from build123d import *

# Parameters (mm, degrees)
SKETCH_3_R      = 3.4
EXTRUDE_1_DEPTH = 2554


with BuildPart() as part:
    # 草图3 → 凸台-拉伸1 (new body)
    with BuildSketch(Plane(origin=(0, 0, 0), x_dir=(1, 0, 0), z_dir=(0, 1, 0))):
        with BuildLine():
            Line((-15, -12.5), (-15, -5.4))
            ThreePointArc((-15, -5.4), (-14.941421356, -5.258578644), (-14.8, -5.2))
            Line((-14.8, -5.2), (-14.4, -5.2))
            ThreePointArc((-14.4, -5.2), (-14.258578644, -5.141421356), (-14.2, -5))
            Line((-14.2, -5), (-14.2, -4.3))
            ThreePointArc((-14.2, -4.3), (-14.141421356, -4.158578644), (-14, -4.1))
            Line((-14, -4.1), (-13.2, -4.1))
            Line((-13.2, -4.1), (-13.2, -8.25))
            Line((-13.2, -8.25), (-9.522792206, -8.25))
            Line((-9.522792206, -8.25), (-5.8, -4.527207794))
            Line((-5.8, -4.527207794), (-5.8, 4.527207794))
            Line((-5.8, 4.527207794), (-9.522792206, 8.25))
            Line((-9.522792206, 8.25), (-13.2, 8.25))
            Line((-13.2, 8.25), (-13.2, 4.1))
            Line((-13.2, 4.1), (-14, 4.1))
            ThreePointArc((-14, 4.1), (-14.141421356, 4.158578644), (-14.2, 4.3))
            Line((-14.2, 4.3), (-14.2, 5))
            ThreePointArc((-14.2, 5), (-14.258578644, 5.141421356), (-14.4, 5.2))
            Line((-14.4, 5.2), (-14.8, 5.2))
            ThreePointArc((-14.8, 5.2), (-14.941421356, 5.258578644), (-15, 5.4))
            Line((-15, 5.4), (-15, 12.5))
            ThreePointArc((-15, 12.5), (-14.267766953, 14.267766953), (-12.5, 15))
            Line((-12.5, 15), (-5.4, 15))
            ThreePointArc((-5.4, 15), (-5.258578644, 14.941421356), (-5.2, 14.8))
            Line((-5.2, 14.8), (-5.2, 14.4))
            ThreePointArc((-5.2, 14.4), (-5.141421356, 14.258578644), (-5, 14.2))
            Line((-5, 14.2), (-4.3, 14.2))
            ThreePointArc((-4.3, 14.2), (-4.158578644, 14.141421356), (-4.1, 14))
            Line((-4.1, 14), (-4.1, 13.2))
            Line((-4.1, 13.2), (-8.25, 13.2))
            Line((-8.25, 13.2), (-8.25, 9.522792206))
            Line((-8.25, 9.522792206), (-4.527207794, 5.8))
            Line((-4.527207794, 5.8), (4.527207794, 5.8))
            Line((4.527207794, 5.8), (8.25, 9.522792206))
            Line((8.25, 9.522792206), (8.25, 13.2))
            Line((8.25, 13.2), (4.1, 13.2))
            Line((4.1, 13.2), (4.1, 14))
            ThreePointArc((4.1, 14), (4.158578644, 14.141421356), (4.3, 14.2))
            Line((4.3, 14.2), (5, 14.2))
            ThreePointArc((5, 14.2), (5.141421356, 14.258578644), (5.2, 14.4))
            Line((5.2, 14.4), (5.2, 14.8))
            ThreePointArc((5.2, 14.8), (5.258578644, 14.941421356), (5.4, 15))
            Line((5.4, 15), (12.5, 15))
            ThreePointArc((12.5, 15), (14.267766953, 14.267766953), (15, 12.5))
            Line((15, 12.5), (15, 5.4))
            ThreePointArc((15, 5.4), (14.941421356, 5.258578644), (14.8, 5.2))
            Line((14.8, 5.2), (14.4, 5.2))
            ThreePointArc((14.4, 5.2), (14.258578644, 5.141421356), (14.2, 5))
            Line((14.2, 5), (14.2, 4.3))
            ThreePointArc((14.2, 4.3), (14.141421356, 4.158578644), (14, 4.1))
            Line((14, 4.1), (13.2, 4.1))
            Line((13.2, 4.1), (13.2, 8.25))
            Line((13.2, 8.25), (9.522792206, 8.25))
            Line((9.522792206, 8.25), (5.8, 4.527207794))
            Line((5.8, 4.527207794), (5.8, -4.527207794))
            Line((5.8, -4.527207794), (9.522792206, -8.25))
            Line((9.522792206, -8.25), (13.2, -8.25))
            Line((13.2, -8.25), (13.2, -4.1))
            Line((13.2, -4.1), (14, -4.1))
            ThreePointArc((14, -4.1), (14.141421356, -4.158578644), (14.2, -4.3))
            Line((14.2, -4.3), (14.2, -5))
            ThreePointArc((14.2, -5), (14.258578644, -5.141421356), (14.4, -5.2))
            Line((14.4, -5.2), (14.8, -5.2))
            ThreePointArc((14.8, -5.2), (14.941421356, -5.258578644), (15, -5.4))
            Line((15, -5.4), (15, -12.5))
            ThreePointArc((15, -12.5), (14.267766953, -14.267766953), (12.5, -15))
            Line((12.5, -15), (5.4, -15))
            ThreePointArc((5.4, -15), (5.258578644, -14.941421356), (5.2, -14.8))
            Line((5.2, -14.8), (5.2, -14.4))
            ThreePointArc((5.2, -14.4), (5.141421356, -14.258578644), (5, -14.2))
            Line((5, -14.2), (4.3, -14.2))
            ThreePointArc((4.3, -14.2), (4.158578644, -14.141421356), (4.1, -14))
            Line((4.1, -14), (4.1, -13.2))
            Line((4.1, -13.2), (8.25, -13.2))
            Line((8.25, -13.2), (8.25, -9.522792206))
            Line((8.25, -9.522792206), (4.527207794, -5.8))
            Line((4.527207794, -5.8), (-4.527207794, -5.8))
            Line((-4.527207794, -5.8), (-8.25, -9.522792206))
            Line((-8.25, -9.522792206), (-8.25, -13.2))
            Line((-8.25, -13.2), (-4.1, -13.2))
            Line((-4.1, -13.2), (-4.1, -14))
            ThreePointArc((-4.1, -14), (-4.158578644, -14.141421356), (-4.3, -14.2))
            Line((-4.3, -14.2), (-5, -14.2))
            ThreePointArc((-5, -14.2), (-5.141421356, -14.258578644), (-5.2, -14.4))
            Line((-5.2, -14.4), (-5.2, -14.8))
            ThreePointArc((-5.2, -14.8), (-5.258578644, -14.941421356), (-5.4, -15))
            Line((-5.4, -15), (-12.5, -15))
            ThreePointArc((-12.5, -15), (-14.267766953, -14.267766953), (-15, -12.5))
        make_face()
        Circle(SKETCH_3_R, mode=Mode.SUBTRACT)
        with BuildLine():
            Line((-13.2, -12.2), (-13.2, -11.05))
            ThreePointArc((-13.2, -11.05), (-12.907106781, -10.342893219), (-12.2, -10.05))
            Line((-12.2, -10.05), (-11.05, -10.05))
            ThreePointArc((-11.05, -10.05), (-10.342893219, -10.342893219), (-10.05, -11.05))
            Line((-10.05, -11.05), (-10.05, -12.2))
            ThreePointArc((-10.05, -12.2), (-10.342893219, -12.907106781), (-11.05, -13.2))
            Line((-11.05, -13.2), (-12.2, -13.2))
            ThreePointArc((-12.2, -13.2), (-12.907106781, -12.907106781), (-13.2, -12.2))
        make_face(mode=Mode.SUBTRACT)
        with BuildLine():
            Line((-10.05, 12.2), (-10.05, 11.05))
            ThreePointArc((-10.05, 11.05), (-10.342893219, 10.342893219), (-11.05, 10.05))
            Line((-11.05, 10.05), (-12.2, 10.05))
            ThreePointArc((-12.2, 10.05), (-12.907106781, 10.342893219), (-13.2, 11.05))
            Line((-13.2, 11.05), (-13.2, 12.2))
            ThreePointArc((-13.2, 12.2), (-12.907106781, 12.907106781), (-12.2, 13.2))
            Line((-12.2, 13.2), (-11.05, 13.2))
            ThreePointArc((-11.05, 13.2), (-10.342893219, 12.907106781), (-10.05, 12.2))
        make_face(mode=Mode.SUBTRACT)
        with BuildLine():
            Line((13.2, 12.2), (13.2, 11.05))
            ThreePointArc((13.2, 11.05), (12.907106781, 10.342893219), (12.2, 10.05))
            Line((12.2, 10.05), (11.05, 10.05))
            ThreePointArc((11.05, 10.05), (10.342893219, 10.342893219), (10.05, 11.05))
            Line((10.05, 11.05), (10.05, 12.2))
            ThreePointArc((10.05, 12.2), (10.342893219, 12.907106781), (11.05, 13.2))
            Line((11.05, 13.2), (12.2, 13.2))
            ThreePointArc((12.2, 13.2), (12.907106781, 12.907106781), (13.2, 12.2))
        make_face(mode=Mode.SUBTRACT)
        with BuildLine():
            Line((10.05, -12.2), (10.05, -11.05))
            ThreePointArc((10.05, -11.05), (10.342893219, -10.342893219), (11.05, -10.05))
            Line((11.05, -10.05), (12.2, -10.05))
            ThreePointArc((12.2, -10.05), (12.907106781, -10.342893219), (13.2, -11.05))
            Line((13.2, -11.05), (13.2, -12.2))
            ThreePointArc((13.2, -12.2), (12.907106781, -12.907106781), (12.2, -13.2))
            Line((12.2, -13.2), (11.05, -13.2))
            ThreePointArc((11.05, -13.2), (10.342893219, -12.907106781), (10.05, -12.2))
        make_face(mode=Mode.SUBTRACT)
    extrude(amount=EXTRUDE_1_DEPTH)


solid = part.part
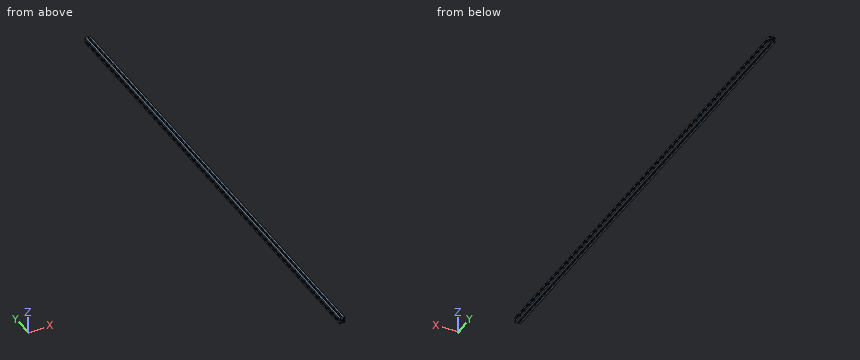
Can you work these out from the model? Positions are in its coordinate system, mm. Round coordinates to 2 decimals unless told otherwise and drop trailing zeros. Write each question's results on one line, items separated by ' | '. Start each with the question number.
1) Please list where these lines run through material, in increasing order: line 1 (Z direction, x = -10.25, y = 1662); line 2 (X direction, y = 791.5, z = 4.5); line 3 (X direction, y = 1025, z = 4.75).
2) For pin 1 Ø0.8 at (y, z) = (674, -4.5) entering from -X; pin 2 Ø5 at (x, z) = (8.5, -0.5) entering from +Y; pin 3 Ø0.9 at (y, z) = (652, -13.5) entering from -X; pin 4 Ø1.5 at (y, z) = (858.5, 1.5) entering from +X, each with a flat end and sliding along its axis, tell me the tip position at first contact or that it passes through.
3) Suppose I cut it at A-A (y = 1233). Give the number of separate pieces and of enclosed holes in the cut face, and give its area (3 significant figures).
Here are the results:
1) line 1: z = -15 to -12.8, -10.45 to -8.25, 8.25 to 10.45, 12.8 to 15 | line 2: x = -14.2 to -13.2, -5.8 to 5.8, 13.2 to 14.2 | line 3: x = -14.2 to -13.2, -6.02 to 6.02, 13.2 to 14.2
2) pin 1: stops at x = -14.2 | pin 2: passes through | pin 3: stops at x = -14.94 | pin 4: stops at x = 5.8
3) separate pieces: 1 | enclosed holes: 5 | area: 323 mm2
